Source: CAD feature listing. Evaluate the final solid. Frame: model axes, mm. A direction names the side the tool comes from. Give positions to 0.01 mm unless a question says otherwise; leave off trailing zeros. Order: outer loops, then holes, each group sorted by start corner. A loop starts at its lowest first (then second) coordinate and runs counter-clockwise, first axis right, second up. Notation, with made-up numbers: (42.25, 31.5) - (93.25, 31.5) arc R21 cw to (93.25, 42.5) - close; hole circle Ø7 at (89, -16). An arc over 180 degrees is marked (long way). Answer as CSV lines item,"result".
```python
from build123d import *

# Parameters (mm, degrees)
ESQUISSE1_W             = 10
ESQUISSE1_H             = 20
ESQUISSE1_R             = 1
BOSS_EXTRU_1_DEPTH      = 2.5
ESQUISSE1_3_W           = 5
ESQUISSE1_3_H           = 2
BOSS_EXTRU_2_DEPTH      = 1.5
BOSS_EXTRU_3_DEPTH      = 1.5
ENL_V_MAT_EXTRU_1_REACH = 26.237
ESQUISSE3_R             = 1
CONG_1_R                = 1
CONG_2_R                = 1


# Read off the part's stored shape, not the designer's step: Révolution1
with BuildPart() as part:
    # Esquisse1 → Boss.-Extru.1 (new, symmetric)
    with BuildSketch(Plane.XY):
        Rectangle(ESQUISSE1_W, ESQUISSE1_H)
        with Locations((2, -5)):
            Circle(ESQUISSE1_R, mode=Mode.SUBTRACT)
        with Locations((2, 5)):
            Circle(ESQUISSE1_R, mode=Mode.SUBTRACT)
    extrude(amount=BOSS_EXTRU_1_DEPTH, both=True)

    # Esquisse1<3> → Boss.-Extru.2 (add, symmetric)
    with BuildSketch(Plane.XY):
        with Locations((7.5, 6.666666667)):
            Rectangle(ESQUISSE1_3_W, ESQUISSE1_3_H)
        with Locations((7.5, 0)):
            Rectangle(ESQUISSE1_3_W, ESQUISSE1_3_H)
        with Locations((7.5, -6.666666667)):
            Rectangle(ESQUISSE1_3_W, ESQUISSE1_3_H)
    extrude(amount=BOSS_EXTRU_2_DEPTH, both=True)

    # Esquisse1<5> → Boss.-Extru.3 (add, symmetric)
    with BuildSketch(Plane.XY):
        Polygon((-5, 9), (-5, 10), (-16.402667816, -9.75), (-15.969655115, -10), align=None)
    extrude(amount=BOSS_EXTRU_3_DEPTH, both=True)

    # Révolution1 outline → Révolution1 (revolve)
    with BuildSketch(Plane(origin=(-8.080127019, 4.665063509, 0), x_dir=(0.8660254037844386, -0.4999999999999999, 0), z_dir=(0, 0, 1))):
        with BuildLine():
            Line((0.5, -14.145081595), (0.5, 3.660254038))
            ThreePointArc((0.5, 3.660254038), (0.35355339, 4.013807428), (0, 4.160254038))
            Line((0, 4.160254038), (0, -14.645081595))
            ThreePointArc((0, -14.645081595), (0.353553391, -14.498634986), (0.5, -14.145081595))
        make_face()
    revolve(axis=Axis((-8.080127019, 4.665063509, 0), (0.4999999999999999, 0.8660254037844386, 0)))

    # Enlèv. mat.-Extru.1: up to this face of the body (flat: up to its plane)
    enl_v_mat_extru_1_end = Plane(part.part.faces().sort_by_distance((7.5, -7.666666667, 0))[0])
    # Esquisse3 → Enlèv. mat.-Extru.1 (cut, up to the picked face)
    with BuildSketch(Plane(origin=(0, 7.666666667, 0), x_dir=(1, 0, 0), z_dir=(0, 1, 0)), mode=Mode.PRIVATE) as enl_v_mat_extru_1_sk1:
        with Locations(Location((7.5, 0, 0), (0, 0, 270))):
            Circle(ESQUISSE3_R)
    enl_v_mat_extru_1_tool1 = split(extrude(enl_v_mat_extru_1_sk1.sketch, amount=-ENL_V_MAT_EXTRU_1_REACH, mode=Mode.PRIVATE), bisect_by=enl_v_mat_extru_1_end, keep=Keep.BOTH, mode=Mode.PRIVATE)
    add(enl_v_mat_extru_1_tool1.solids().sort_by(Axis((7.5, 7.666667, 0), (0, -1, 0)))[0], mode=Mode.SUBTRACT)

    # Congé1
    cong_1_edges = [part.edges().sort_by_distance(p)[0] for p in [
        (5, -10, 0),
        (-5, -10, 0),
        (5, 10, 0),
        (-16.186161466, -9.875, -1.5),
        (-16.186161466, -9.875, 1.5),
    ]]
    fillet(cong_1_edges, radius=CONG_1_R)

    # Congé2
    cong_2_edges = [part.edges().sort_by_distance(p)[0] for p in [
        (10, 6.666666667, 1.5),
        (10, 6.666666667, -1.5),
        (10, 0, 1.5),
        (10, 0, -1.5),
        (10, -6.666666667, -1.5),
        (10, -6.666666667, 1.5),
    ]]
    fillet(cong_2_edges, radius=CONG_2_R)


solid = part.part
```
(1) Cut plane C-C (z = -1.95). Return loops of the section in (x, y).
Completed:
outline,"(-5, -9) arc R1 ccw to (-4, -10) - (4, -10) arc R1 ccw to (5, -9) - (5, 9) arc R1 ccw to (4, 10) - (-5, 10) - close; hole circle Ø2 at (2, -5); hole circle Ø2 at (2, 5)"
(2) Cut plane B-B (x = 2). Return loops of the section in (y, z).
Completed:
outline,"(-10, -2.5) - (-6, -2.5) - (-6, 2.5) - (-10, 2.5) - close; (-4, -2.5) - (4, -2.5) - (4, 2.5) - (-4, 2.5) - close; (6, -2.5) - (10, -2.5) - (10, 2.5) - (6, 2.5) - close"
(3) Cut plane A-A (x = 7.5). Return loops of the section in (y, z), then the cut area to 3 significant figures.
Completed:
outline,"(-7.67, -1.5) - (-5.67, -1.5) - (-5.67, -1) - (-7.67, -1) - close; (-7.67, 1) - (-5.67, 1) - (-5.67, 1.5) - (-7.67, 1.5) - close; (-1, -1.5) - (1, -1.5) - (1, -1) - (-1, -1) - close; (-1, 1) - (1, 1) - (1, 1.5) - (-1, 1.5) - close; (5.67, -1.5) - (7.67, -1.5) - (7.67, -1) - (5.67, -1) - close; (5.67, 1) - (7.67, 1) - (7.67, 1.5) - (5.67, 1.5) - close"
area,"6.00 mm²"
(4) Access query for faces 1 (the cylindrical face through (9.699, -6.653, 1.215)), 2 (the flat face through (6, -1, 0)), 3 (the flat face through (0, -10, 0)), 4 (the flat face through (-11, -1, 1.5)), 5 (the flat face through (7, -7, -1.5)). Directions: +Z, -Z, +X, -X, +Y, -Y. A direction counts if a zero-diameter tool reaches every point of the face in a straight line with its end or side. Return the directions, or none.
Completed:
face 1,"+Z, +X, +Y, -Y"
face 2,"+Z, -Z, +X"
face 3,"+Z, -Z, +X, -X, -Y"
face 4,"+Z, -X, +Y, -Y"
face 5,"-Z, +X, +Y, -Y"
(5) Mould query, pull axis Y, two halves, no side actions, for faces 6 (the flat face through (-5, 0, 0)), 7 (the flat face through (6, 7.667, 0)), 8 (the flat face through (6, 1, 0)). Classes: released by +Y, released by -Y, zero draft, split by the parting line, or undercut.
Completed:
face 6,"zero draft"
face 7,"released by +Y"
face 8,"undercut"
(6) Cut plane D-D (y = -5). Give the number of separate pieces and of enclosed holes in the cut face, then the cut area to 3 significant figures.
Completed:
separate pieces,"3"
enclosed holes,"0"
area,"42.2 mm²"
(7) Ray query, line 1 (Y direction, x = 2, z = -0.5); line 2 (Y direction, x = 5.75, z = 0.5); line 3 (X direction, y = -6.8, z = 0). Return the intervals inside material, ascending. Write a range as from..to.
Completed:
line 1,"-10..-6, -4..4, 6..10"
line 2,"-7.67..-5.67, -1..1, 5.67..7.67"
line 3,"-15.28..-14.12, -5..6.5, 8.5..10"
(8) Contact query for flat-ended pins moving along their axis: pin 1 (1.2 mm diameter, centred on x = 7.5, z = 0, fed in from -Y); pin 2 (2.5 mm diameter, centred on x = 8.5, z = 0.5, fed in from -Y); pin 3 (2 mm diameter, centred on y = -3, z = 0.5, fed in from -X); pin 4 (1.5 mm diameter, centred on y = -6, z = -1.5, fed in from +X). Output: stop coordinate, or through.
Completed:
pin 1,"through"
pin 2,"y = -7.67"
pin 3,"x = -13.6"
pin 4,"x = 9.97"
